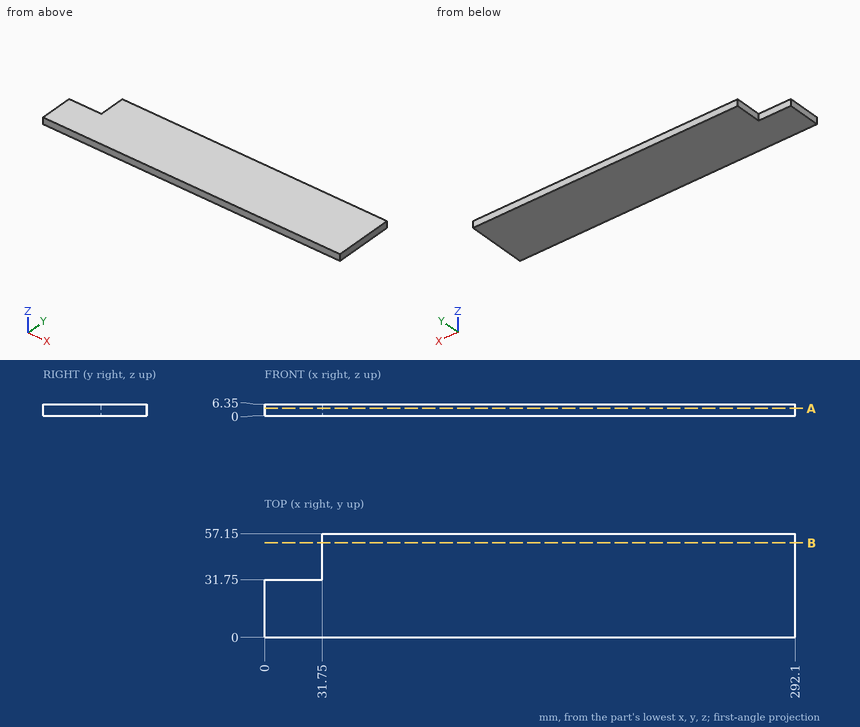
Geometry check sheet. Reference: drawing and pictorial views, mm from the part's lowest x, y, z. Round coordinates to 2 decimals unless told otherwise and drop trailing zeros. Order: outer loops, then holes, each group sorted by start corner. A loop starts at its lowest first (then second) coordinate and runs counter-clockwise, first axis right, second up. Notation, with made-up numbers: (86.5, -16) - (140.5, -16) arc R11 cw to (140.5, -2) - close; hole circle Ø1 at (66, -29.5). An arc over 180 degrees is marked (long way). One line per question, with ' | ' between items. Start each with the question number.
(1) Sectioned sample at A-A on z = 4. Record the cut outline in (x, y), and give its area (3 significant figures).
(2) Thickness scan on L1, parallel to X at y = 52, z = 2.5; L2, parallel to Y at x = 19, z = 0.5. Record the ranges inside material, lowest first. Write a range as [from, to].
(3) Sectioned sample at B-B on y = 52. Record the cut outline in (x, z).
(4) Depth check by flat-ended pin: pin 1 Ø2 at (y, z) = (50, 5.5) entering from -X; pin 2 Ø2 at (x, y) = (194.5, 50.5) entering from -Z. Enter the tip coordinate at first touch or a pass-through.
Conclusion:
1) outline: (0, 0) - (292.1, 0) - (292.1, 57.15) - (31.75, 57.15) - (31.75, 31.75) - (0, 31.75) - close | area: 15,900 mm2
2) L1: x = [31.75, 292.1] | L2: y = [0, 31.75]
3) outline: (31.75, 0) - (292.1, 0) - (292.1, 6.35) - (31.75, 6.35) - close
4) pin 1: stops at x = 31.75 | pin 2: stops at z = 0
